Solid Edge part; units mm, degrees
sketch "Sketch1" plane through (0, 0, 0) normal (0, -1, 0) x (1, 0, 0)
  line L0 (0, 2) -> (0, 0)
  line L1 (0, 0) -> (6, 0)
  line L2 (9, 2.5) -> (6, 0)
  line L3 (6, 2.5) -> (9, 2.5)
  line L4 (6, 2.5) -> (2, 2.5)
  line L5 (2, 2.5) -> (2, 2)
  line L6 (2, 2) -> (0, 2)
revolve "RevolvedProtrusion1" add sketch "Sketch1" angle 360 about axis through (6, 0, 2.5) along (1, 0, 0)
chamfer "Chanfro_1" distance 0.26 angle 45 1 edges at (0, 0, 5) measured on face at (0, -1.6167, 0.7833)
sketch "Sketch2" plane through (0, 0, 2.5) normal (-1, 0, 0) x (0, -1, 0)
  line L0 (0.5, 2.4495) -> (0.5, 0)
  line L1 (0.5, 0) -> (0.5, -2.4495)
  arc A0 (0.5, -2.4495) -> (-0.5, -2.4495) centre (0, 0) cw
  line L2 (-0.5, 0) -> (-0.5, -2.4495)
  line L3 (-0.5, 0) -> (-0.5, 2.4495)
  arc A1 (-0.5, 2.4495) -> (0.5, 2.4495) centre (0, 0) cw
extrude "Recorte_Extrudado_1" cut sketch "Sketch2" against normal blind 2
The model under review builds one solid part; all positions refer to its coordinate system, in mm. Round coordinates to 2 decimals unless told otherwise and drop trailing zeros. Write each loop counter-clockwise with the first axis right and the second up, starting at its lowest first coordinate (ties: lowest second). Pieces come first, ordered by that corner, then holes. Notation, with made-up numbers: (3, 64) - (9, 64) arc R21 cw to (9, 92) - close; hole circle Ø1 at (20.25, 43). An arc over 180 degrees is marked (long way). One line per item, written item: value. Start each with the question number.
1. To check wall thickness, follow L1, parallel to Y at x = 1, z = 2.6; L2, parallel to Y at x = 1.5, z = 1.2; L3, parallel to Z at x = 3, y = -0.1. State the ranges of each line that lie inside material, in increasing order. Write a range as from..to.
2. Consider section A-A on x = 0.5. Write out the cut boundary in (y, z), and give its area (3 significant figures).
3. Clearance check with flat-ended pins moving along their axes: P1, Ø1.6, axis at x = 1, z = 1, coming from the +Y side; P2, Ø0.5, axis at y = 0, z = 3, coming from the -X side; P3, Ø1, axis at x = 1, z = 3.5, coming from the -Y side. State where each tip first meets the part, or that it passes through.
4. Consider section C-C on x = 6.75. Write out the cut boundary in (y, z) (3 decimals), and give its area (3 significant figures).
5. The part is to be moulded in two halves that separate along Y. For faces 1 (the face through (2, 0, 2)), 2 (the face through (0, 1, 3)), 3 (the face through (0.13, 2.37, 2.45)), say which applies: released by +Y, released by -Y, zero draft, split by the parting line, or undercut.
6. Consider section B-B on x = 5. Write out the cut boundary in (y, z), and give its area (3 significant figures).
Checks:
1. L1: y = -2.5..-0.5, 0.5..2.5
1. L2: y = -2.14..-0.5, 0.5..2.14
1. L3: z = 0..5
2. outline: (-0.5, 0.05) - (-0.5, 2.5) - (-0.5, 4.95) arc R2.5 ccw to start; (0.5, 0.05) arc R2.5 ccw to (0.5, 4.95) - (0.5, 2.5) - close
2. area: 14.7 mm^2
3. P1: stops at y = 2.4
3. P2: stops at x = 2
3. P3: stops at y = -2.45
4. outline: circle Ø3.75 at (0, 2.5)
4. area: 11.0 mm^2
5. face 1: undercut
5. face 2: zero draft
5. face 3: released by +Y
6. outline: circle Ø5 at (0, 2.5)
6. area: 19.6 mm^2
